Work out the finished part from the listing and answer in its coordinate system (mm). Round coordinates to 2 decimals unless told otherwise and drop trailing zeros. Loops run counter-clockwise (first coordinate to the right, second up) from the corner with the lowest first, then second, coordinate; pieces in that order, holes last. Notation, with made-up numbers: (54, 74) - (88, 74) arc R9 ccw to (88, 82) - close; hole circle Ø2 at (-39.75, -18.75). An arc over 180 degrees is marked (long way). Answer as CSV lines item,"result". Start each with the question number.
Q1. Section B-B on z = 58.5 is taken. Write down the section's boundary in (x, y), then the cut area to 3 significant figures.
Q2. Straight lines are drawn through the part: L1, parallel to Y at x = 1.5, z = 39; L2, parallel to Z at x = 0.3, y = 11; L3, parallel to Z at x = 0.75, y = 13.5. For each, find the intervals that lie inside material, in ascending order. Write a range as [from, to].
Q3. Section C-C on y = -20.5 is taken. Write down the section's boundary in (x, z).
Q4. The mould has two halves that part along Z. Classify faces 1 (the face through (1.521, 0.55, -24.994)), 2 (the face through (3, 5, 89)), 3 (the face through (2, 0, 178)): +Z half, -Z half, draft (parallel to the pull), parting line (faces both ways), or undercut.
Q5. Section A-A on x = 1.5 is taken. Write down the section's boundary in (y, z).
```python
from build123d import *

# Parameters (mm, degrees)
F0_W        = 50
F0_H        = 400
F1_DEPTH    = 3
F2_T1_DEPTH = 128
F3_R        = 3
F4_DEPTH    = 25
F6_DEPTH    = 25
F8_DEPTH    = 25


# Not quite as in the source:
# - a fillet or chamfer that OpenCascade refuses, or shapes differently, is made with other operations: its cross-section is extruded or revolved along the edge and cut away or added


with BuildPart() as f1:
    # F0 (on Right) → F1 (new body)
    with BuildSketch(Plane.YZ):
        Rectangle(F0_W, F0_H)
    extrude(amount=F1_DEPTH)

    # F2: fillet of radius 25 on 4 edges, made by hand

    # F2_s2 → F2_t1 (cut)
    with BuildSketch(Plane.YZ.offset(-62.5)):
        with BuildLine():
            ThreePointArc((0, 200), (-17.6776695297, 192.6776695297), (-25, 175))
            Line((-25, 175), (-25, 200))
            Line((-25, 200), (0, 200))
        make_face()
        with BuildLine():
            ThreePointArc((-25, -175), (-17.6776695297, -192.6776695297), (0, -200))
            Line((0, -200), (-25, -200))
            Line((-25, -200), (-25, -175))
        make_face()
        with BuildLine():
            ThreePointArc((25, 175), (17.6776695297, 192.6776695297), (0, 200))
            Line((0, 200), (25, 200))
            Line((25, 200), (25, 175))
        make_face()
        with BuildLine():
            ThreePointArc((25, -175), (17.6776695297, -192.6776695297), (0, -200))
            Line((0, -200), (25, -200))
            Line((25, -200), (25, -175))
        make_face()
    extrude(amount=F2_T1_DEPTH, mode=Mode.SUBTRACT)

    # F3 (on face) → F4 (cut)
    with BuildSketch(Plane.YZ.offset(3)):
        with Locations((0, 175)):
            Circle(F3_R)
    extrude(amount=-F4_DEPTH, mode=Mode.SUBTRACT)

    # F5 (on face) → F6 (cut)
    with BuildSketch(Plane.YZ.offset(3)):
        with BuildLine():
            ThreePointArc((-3, 100), (0, 97), (3, 100))
            ThreePointArc((3, 100), (0, 103), (-3, 100))
        make_face()
        with BuildLine():
            Line((3, 0), (3, 100))
            ThreePointArc((3, 100), (0, 97), (-3, 100))
            Line((-3, 100), (-3, 0))
            ThreePointArc((-3, 0), (0, 3), (3, 0))
        make_face()
        with BuildLine():
            ThreePointArc((-3, 0), (0, -3), (3, 0))
            ThreePointArc((3, 0), (0, 3), (-3, 0))
        make_face()
    extrude(amount=-F6_DEPTH, mode=Mode.SUBTRACT)

    # F7 (on face) → F8 (cut)
    with BuildSketch(Plane.YZ.offset(3)):
        with BuildLine():
            ThreePointArc((25, 0), (0, -25), (-25, 0))
            Line((-25, 0), (-25, -175))
            ThreePointArc((-25, -175), (0, -200), (25, -175))
            Line((25, -175), (25, 0))
        make_face()
    extrude(amount=-F8_DEPTH, mode=Mode.SUBTRACT)


solid = f1.part
```
Findings:
1,outline,"(0, -25) - (3, -25) - (3, -3) - (0, -3) - close; (0, 3) - (3, 3) - (3, 25) - (0, 25) - close"
1,area,"132 mm^2"
2,L1,"y = [-25, -3], [3, 25]"
2,L2,"z = [-22.45, 197.45]"
2,L3,"z = [-21.04, 196.04]"
3,outline,"(0, -14.31) - (3, -14.31) - (3, 189.31) - (0, 189.31) - close"
4,face 1,"-Z half"
4,face 2,"draft"
4,face 3,"undercut"
5,outline,"(-25, 0) arc R25 ccw to (25, 0) - (25, 175) arc R25 ccw to (-25, 175) - close; hole (-3, 0) arc R3 ccw to (3, 0) - (3, 100) arc R3 ccw to (-3, 100) - close; hole circle Ø6 at (0, 175)"
